```python
from build123d import *

# Parameters (mm, degrees)
F0_R     = 22.766123
F1_DEPTH = 13.56037
F2_R     = 42.909984
F2_R_2   = 22.766123
F3_DEPTH = 69.79863
F4_R     = 17.01771
F5_DEPTH = 13.11468
F6_R     = 15.24
F8_D     = 25.4


with BuildPart() as f1:
    # F0 (on Top) → F1 (new body)
    with BuildSketch(Plane.XY):
        Circle(F0_R)
    extrude(amount=F1_DEPTH)

    # F2 (on face) → F3 (join)
    with BuildSketch(Plane.XY.offset(13.56037)):
        Circle(F2_R)
        Circle(F2_R_2, mode=Mode.SUBTRACT)
        Circle(F2_R_2)
    extrude(amount=F3_DEPTH)

    # F4 (on face) → F5 (join)
    with BuildSketch(Plane.XY.offset(83.359)):
        Circle(F4_R)
    extrude(amount=F5_DEPTH)

    # F6
    f6_edges = [f1.edges().sort_by_distance(p)[0] for p in [
        (-42.909984, 0, 83.359),
        (-42.909984, 0, 13.56037),
    ]]
    fillet(f6_edges, radius=F6_R)

    # F8 (through all)
    with Locations(Plane.XY.offset(96.47368)):
        with Locations((0, 0)):
            Hole(F8_D / 2)


solid = f1.part
```
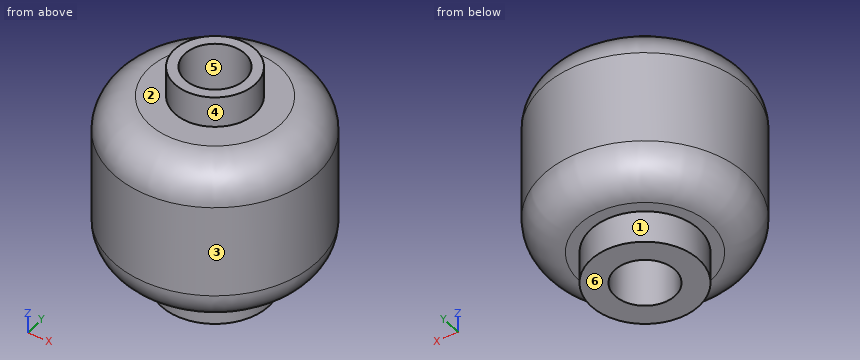
Input: part model. Units: mm. Frame: model coordinates. Face numbers are marked on the shaded views. A direction names the side the tool comes from. Round coordinates to 2 decimals unless told otherwise and drop trailing zeros. Loops run counter-clockwise (first coordinate to the right, second up) from the corner with the lowest first, then second, coordinate; pieces in that order, holes last. Notation, with made-up numbers: (-18.5, -8) -> (-0.5, -8) arc R27 ccw to (-0.5, 22) -> close; hole circle Ø7 at (62.25, -16). An arc over 180 degrees is marked (long way). Write each question's results on one line, items separated by ' | '.
1. Set-up query: the marked faces 1, 2 and 3. Return all of +Z, -Z, +X, -X, +Y, -Y with unobstructed straight access to the full face (end or side cutting, diameter ignored); none if empty.
Geometry results:
face 1: -Z | face 2: +Z | face 3: +Z, -Z
2. Mould query, pull axis Y, two halves, no side actions, for the marked faces 4, 5 and 6. Classes: +Y half, -Y half, draft (parallel to the pull), parting line (faces both ways), or undercut.
Geometry results:
face 4: parting line | face 5: undercut | face 6: draft
3. Section A-A (x = 0). Return loops of the section in (y, z), and give its area (3 significant figures).
Geometry results:
outline: (-42.91, 28.8) arc R15.24 ccw to (-27.67, 13.56) -> (-22.77, 13.56) -> (-22.77, 0) -> (-12.7, 0) -> (-12.7, 96.47) -> (-17.02, 96.47) -> (-17.02, 83.36) -> (-27.67, 83.36) arc R15.24 ccw to (-42.91, 68.12) -> close; (12.7, 0) -> (22.77, 0) -> (22.77, 13.56) -> (27.67, 13.56) arc R15.24 ccw to (42.91, 28.8) -> (42.91, 68.12) arc R15.24 ccw to (27.67, 83.36) -> (17.02, 83.36) -> (17.02, 96.47) -> (12.7, 96.47) -> close | area: 4,400 mm2
4. First-contact query: P1, Ø8, axis at y = -30.5, z = 45, coming from the -X side; P2, Ø1, axis at x = 10.5, z = 57.5, coming from the -Y side; P3, Ø4, axis at x = 27, z = 61, coming from the +Y side (3 decimals). Flat tips, straight axial feed; report the tip coordinate or a pass-through.
Geometry results:
P1: x = -33.75 | P2: y = -41.73 | P3: y = 34.875
5. Section C-C (z = 43.5). Return loops of the section in (x, y), and give its area (3 significant figures).
Geometry results:
outline: circle Ø85.82 at (0, 0); hole circle Ø25.4 at (0, 0) | area: 5,280 mm2
6. Ray query, line 1 (Z direction, x = -22, y = -5); line 2 (Z direction, x = 17, y = -18.5); line 3 (X direction, y = -3.5, z = 35). Return the intervals inside material, ascending. Write a range as from..to.
Geometry results:
line 1: 0..83.36 | line 2: 13.56..83.36 | line 3: -42.77..-12.21, 12.21..42.77
7. Section D-D (z = 25). Return loops of the section in (x, y).
Geometry results:
outline: circle Ø84.86 at (0, 0); hole circle Ø25.4 at (0, 0)
